Source: CAD feature listing. Evaluate the final solid. Frame: model axes, mm. A direction names the side the tool comes from. Coordinates: 2 decimals unless noted, no trailing zeros. Write each loop counter-clockwise with the first axis right and the second up, starting at its lowest first coordinate (ties: lowest second). Pieces come first, ordered by that corner, then holes. Notation, with made-up numbers: (66.25, 72.25) - (118.25, 72.25) arc R21 cw to (118.25, 103.25) - close; hole circle Ø2 at (-34, 27). An arc over 180 degrees is marked (long way). One line per item, written item: value.
from build123d import *

# Parameters (mm, degrees)
SKETCH1_R           = 1.35
SKETCH1_W           = 6
SKETCH1_H           = 38.1
SKETCH1_H_2         = 6
BOSS_EXTRUDE1_DEPTH = 3
FILLET1_R           = 2.54
CUT_EXTRUDE1_DEPTH  = 81.055232476
LPATTERN1_COUNT     = 2
LPATTERN1_PITCH     = 12.7
SKETCH3_W           = 2.75
SKETCH3_H           = 6.096
CUT_EXTRUDE2_DEPTH  = 81.055232476
LPATTERN2_COUNT     = 3
LPATTERN2_PITCH     = 12.7


with BuildPart() as part:
    # Sketch1 → Boss-Extrude1 (new, symmetric)
    # profile 1 of 3: a face of its own
    with BuildSketch(Plane.XY):
        with BuildLine():
            Line((-62.999206449, -30.043127024), (-50.388789218, -3))
            Line((-50.388789218, -3), (49.3, -3))
            Line((49.3, -3), (49.3, 3))
            Line((49.3, 3), (-52.3, 3))
            ThreePointArc((-52.3, 3), (-53.911898825, 2.530174337), (-55.018923361, 1.267854785))
            Line((-55.018923361, 1.267854785), (-55.3, 0.665083988))
            Line((-55.3, 0.665083988), (-68.437053171, -27.507417453))
            Line((-68.437053171, -27.507417453), (-62.999206449, -30.043127024))
        make_face()
        with Locations((-52.3, 0)):
            Circle(SKETCH1_R, mode=Mode.SUBTRACT)
    # profile 2 of 3: a face of its own
    with BuildSketch(Plane.XY):
        with Locations((52.3, -22.05)):
            Rectangle(SKETCH1_W, SKETCH1_H)
    # profile 3 of 3: a face of its own
    with BuildSketch(Plane.XY):
        with Locations((52.3, 0)):
            Rectangle(SKETCH1_W, SKETCH1_H_2)
    extrude(amount=BOSS_EXTRUDE1_DEPTH, both=True)

    # Fillet1
    fillet1_edges = [part.edges().sort_by_distance(p)[0] for p in [
        (-50.388789218, -3, 0),
    ]]
    fillet(fillet1_edges, radius=FILLET1_R)

    # Sketch2 → Cut-Extrude1 (cut, symmetric)
    with BuildSketch(Plane.XY.offset(3)):
        Polygon((-63.046209113, -19.791792635), (-65.622490036, -25.316644905), (-63.130143622, -26.478845124), (-60.553862698, -20.953992855), align=None)
    cut_extrude1 = extrude(amount=CUT_EXTRUDE1_DEPTH, both=True, mode=Mode.SUBTRACT)

    # LPattern1: Cut-Extrude1 ×2
    with Locations(*[Vector(0.42261826174070405, 0.9063077870366479, 0) * (i * LPATTERN1_PITCH) for i in range(1, LPATTERN1_COUNT)]):
        add(cut_extrude1, mode=Mode.SUBTRACT)

    # Sketch3 → Cut-Extrude2 (cut, symmetric)
    with BuildSketch(Plane.XY.offset(3)):
        with Locations((52.3, -31.702)):
            Rectangle(SKETCH3_W, SKETCH3_H)
    cut_extrude2 = extrude(amount=CUT_EXTRUDE2_DEPTH, both=True, mode=Mode.SUBTRACT)

    # LPattern2: Cut-Extrude2 ×3
    with Locations(*[(0, i * LPATTERN2_PITCH, 0) for i in range(1, LPATTERN2_COUNT)]):
        add(cut_extrude2, mode=Mode.SUBTRACT)


solid = part.part
1) Contact query for flat-ended pins moving along their axis: P1, Ø1.8, axis at y = -6.5, z = -1, coming from the -X side; P2, Ø3, axis at y = -18, z = 0.5, coming from the -X side. Output: stop coordinate, or through.
Values found:
P1: x = -59.06
P2: x = -64.7
2) Reachability of faces 4 (the flat face through (49.3, -22, 0)), 5 (the flat face through (-2.3, -2.6, 3)), 6 (the flat face through (-56.49, -12.24, 0.04)) from +Z, -Z, +X, -X, +Y, -Y: full face, straight path, thin tool, end or side. Return the list, or none.
Values found:
face 4: +Z, -Z, -Y
face 5: +Z, +X, -X, +Y, -Y
face 6: +Z, -Z
3) Section query C-C on x = -4. Output: boundary loops of the cut face in (y, z), then the cut area to 3 significant figures.
Values found:
outline: (-3, -3) - (3, -3) - (3, 3) - (-3, 3) - close
area: 36.0 mm2
4) Section query B-B on y = -11. Output: boundary loops of the cut face in (x, z).
Values found:
outline: (-60.74, -3) - (-58.95, -3) - (-58.95, 3) - (-60.74, 3) - close; (-55.91, -3) - (-54.12, -3) - (-54.12, 3) - (-55.91, 3) - close; (49.3, -3) - (55.3, -3) - (55.3, 3) - (49.3, 3) - close
5) Material intervals for line 1 (X direction, y = -12, z = -1.5); line 2 (X direction, y = -22, z = 1.45) (3 decimals); line 3 (X direction, y = -34.5, z = -2.2) (3 decimals), sorted ascending.
Values found:
line 1: -61.21 to -59.41, -56.38 to -54.59, 49.3 to 55.3
line 2: -65.869 to -64.076, -61.042 to -59.249, 49.3 to 50.925, 53.675 to 55.3
line 3: 49.3 to 50.925, 53.675 to 55.3
6) Draft query along X for faces 1 (the flat face through (52, -41.1, 0)), 2 (the flat face through (-65.756, -28.758, 0.042)), 3 (the flat face through (53.675, -19, 0)). Return one class per face: released by +X, released by -X, zero draft, split by the parting line, or undercut.
Values found:
face 1: zero draft
face 2: released by -X
face 3: undercut
7) Section query A-A on z = 1.25. State how many separate pieces and enclosed holes the cut face has, then the cut area to 3 significant figures.
Values found:
separate pieces: 1
enclosed holes: 6
area: 975 mm2
